Geometry check sheet. Reference: the model listing, model coordinates, mm. A direction names the side the tool comes from. Round coordinates to 2 decimals unless told otherwise and drop trailing zeros. Order: outer loops, then holes, each group sorted by start corner. A loop starts at its lowest first (then second) coordinate and runs counter-clockwise, first axis right, second up. Notation, with made-up numbers: (-26.75, 62.25) - (10.25, 62.25) arc R10 cw to (10.25, 78.25) - close; hole circle Ø8 at (71, 17.25). An arc over 180 degrees is marked (long way). Use a Markdown table: item, result. Add a question column.
(1) Gauge pin test, flat ends, axial feed: P1, Ø1.5, axis at x = 126, y = -13, coming from the +Z side; P2, Ø2, axis at y = -35, z = 22.5, coming from the -X side. Record the tip position at first contact, or that the pin passes through.
(2) Section check A-A on x = 16. Record the boundary of the cut face in (y, z).
(3) Access from +Z, -Z, +X, -X, +Y, -Y to the whole of each face (thin tool, end or side, straight path). Record for faces 1 (the face through (131, -38, 27.023)), 2 (the face through (108, -7.229, 20)).
(4) Section check B-B on z = 17. Record the boundary of the cut face in (x, y), then the cut area to 3 significant figures.
(5) Thickness scan on line 1 along Y through (x, z) = (162, 26); line 2 along Z through (x, y) = (34, -29); line 3 along X through (y, z) = (-30.5, 17.25). Record the ranges inside material, lowest first. Write a range as [from, to].
(6) Mould release check, pull along Y, two halves, no side actions. Record for faces 3 (the face through (113, -3.419, 17)), 4 (the face through (108, -37.709, 20)), 5 (the face through (228.6, -23, 17)): released by +Y, released by -Y, zero draft, split by the parting line, or undercut.
(7) Section check C-C on y = -35. Record the boundary of the cut face in (x, z), then the cut area to 3 significant figures.
```python
from build123d import *

# Parameters (mm, degrees)
F1_DEPTH = 228.6
F2_DEPTH = 228.6
F3_W     = 10.16
F3_H     = 30.48
F4_DEPTH = 13.97


with BuildPart() as f1:
    # F0 (on Right) → F1 (new body)
    with BuildSketch(Plane.YZ):
        Polygon((-41.518882, 27.023025), (-41.518882, 7.973025), (-3.418882, 7.973025), (-3.418882, 27.023025), (-7.228882, 27.023025), (-7.228882, 13.053025), (-37.708882, 13.053025), (-37.708882, 27.023025), align=None)
    extrude(amount=F1_DEPTH)

    # F0 (on Right) → F2 (join)
    with BuildSketch(Plane.YZ):
        Polygon((-41.518882, 27.023025), (-41.518882, 7.973025), (-3.418882, 7.973025), (-3.418882, 27.023025), (-7.228882, 27.023025), (-7.228882, 13.053025), (-37.708882, 13.053025), (-37.708882, 27.023025), align=None)
    extrude(amount=F2_DEPTH)

    # F3 (on face) → F4 (join)
    with BuildSketch(Plane.XY.offset(13.053025)):
        with Locations((223.52, -22.468882)):
            Rectangle(F3_W, F3_H)
    extrude(amount=F4_DEPTH)


with BuildPart() as f5_1:
    # F5: copy of F1
    add(f1.part)


solid = f1.part
```
Check sheet entries:
| question | item | result |
|---|---|---|
| 1 | P1 | stops at z = 13.05 |
| 1 | P2 | stops at x = 218.44 |
| 2 | outline | (-41.52, 7.97) - (-3.42, 7.97) - (-3.42, 27.02) - (-7.23, 27.02) - (-7.23, 13.05) - (-37.71, 13.05) - (-37.71, 27.02) - (-41.52, 27.02) - close |
| 3 | face 1 | +Z, +X, -X, +Y, -Y |
| 3 | face 2 | +Z, -X |
| 4 | outline | (0, -41.52) - (228.6, -41.52) - (228.6, -3.42) - (0, -3.42) - (0, -7.23) - (218.44, -7.23) - (218.44, -37.71) - (0, -37.71) - close |
| 4 | area | 2,050 mm2 |
| 5 | line 1 | y = [-41.52, -37.71], [-7.23, -3.42] |
| 5 | line 2 | z = [7.97, 13.05] |
| 5 | line 3 | x = [218.44, 228.6] |
| 6 | face 3 | released by +Y |
| 6 | face 4 | undercut |
| 6 | face 5 | zero draft |
| 7 | outline | (0, 7.97) - (228.6, 7.97) - (228.6, 27.02) - (218.44, 27.02) - (218.44, 13.05) - (0, 13.05) - close |
| 7 | area | 1,300 mm2 |
